```python
from build123d import *

# Parameters (mm, degrees)
SKETCH2_R          = 4
SKETCH2_R_2        = 1.75
CUT_EXTRUDE1_DEPTH = 21.310096012


with BuildPart() as part:
    # Sketch1 → Revolve1 (revolve)
    with BuildSketch(Plane.XY, mode=Mode.PRIVATE) as revolve1_sk:
        Polygon((0, 0), (12.5, 0), (12.5, -4), (6.5, -4), (6.5, -10), (0, -10), align=None)
    revolve(revolve1_sk.sketch.rotate(Axis((0, -10, 0), (0, 1, 0)), 90), axis=Axis((0, -10, 0), (0, 1, 0)))

    # Sketch2 → Cut-Extrude1 (cut, through all)
    with BuildSketch(Plane(origin=(0, 0, 0), x_dir=(1, 0, 0), z_dir=(0, 1, 0))):
        with Locations(Location((0, 0, 0), (0, 0, 270))):
            Circle(SKETCH2_R)
        with Locations(Location((0, 9.5, 0), (0, 0, 270))):
            Circle(SKETCH2_R_2)
        with Locations(Location((9.5, 0, 0), (0, 0, 270))):
            Circle(SKETCH2_R_2)
        with Locations(Location((0, -9.5, 0), (0, 0, 270))):
            Circle(SKETCH2_R_2)
        with Locations(Location((-9.5, 0, 0), (0, 0, 270))):
            Circle(SKETCH2_R_2)
    extrude(amount=-CUT_EXTRUDE1_DEPTH, mode=Mode.SUBTRACT)


solid = part.part
```
Check sheet for the modelled part. Datum: model origin and axes. Units: mm. A direction names the side the tool comes from. Give positions to 0.01 mm unless a question says otherwise; leave off trailing zeros. Order: outer loops, then holes, each group sorted by start corner. A loop starts at its lowest first (then second) coordinate and runs counter-clockwise, first axis right, second up. Notation, with made-up numbers: M -18,11.5 L 36,11.5 A9 cw 36,16.5 Z; hole C 72,15 d4. An arc over 180 degrees is marked long. Answer in a Markdown table with one row per item. Add a question column.
Q1. Sectioned sample at D-D, the plane z = -9.5. Record the boundary of the cut face in (x, y), and give its area (3 significant figures).
Q2. Sectioned sample at A-A, the plane x = 0. Record the boundary of the cut face in (y, z), and give its area (3 significant figures).
Q3. Thickness scan on L1, parallel to X at y = -0.25, z = 0; L2, parallel to X at y = -8, z = -0.25; L3, parallel to Y at x = 9.25, z = 3.25. Record the ranges inside material, lowest first.
Q4. Sectioned sample at C-C, the plane x = 10.25. Record the boundary of the cut face in (y, z).
Q5. Gauge pin test, flat ends, axial feed: pin 1 Ø5 at (y, z) = (-4.5, -5) entering from +X; pin 2 Ø5 at (x, z) = (0, 0) entering from -Y (3 decimals); pin 3 Ø4.5 at (x, z) = (0, 9.5) entering from -Y; pin 4 Ø5 at (x, y) = (-5, -5.5) entering from +Z. Record the tip position at first contact, or that the pin passes through.
Q6. Release check for a two-part mould opening along Z. For faces 1 (the cylindrical face through (-3.755, -2.028, -11.923)), 2 (the cylindrical face through (-3.905, -4.93, -0.867)), 3 (the flat face through (-3, -10, -3)) record: released by +Z, released by -Z, zero draft, split by the parting line, or undercut.
Q7. Sectioned sample at B-B, the plane z = 0. Record the boundary of the cut face in (x, y).
Q8. Access from +Z, -Z, +X, -X, +Y, -Y to the whole of each face (thin tool, end or side, straight path). Record for faces 4 (the cylindrical face through (0.526, -1.972, 11.169)), 5 (the cylindrical face through (3.955, -7.042, 5.158)).
Verdict:
| question | item | result |
|---|---|---|
| 1 | outline | M -8.12,-4 L -1.75,-4 L -1.75,0 L -8.12,0 Z; M 1.75,-4 L 8.12,-4 L 8.12,0 L 1.75,0 Z |
| 1 | area | 51.0 mm² |
| 2 | outline | M -10,-6.5 L -4,-6.5 L -4,-7.75 L 0,-7.75 L 0,-4 L -10,-4 Z; M -10,4 L 0,4 L 0,7.75 L -4,7.75 L -4,6.5 L -10,6.5 Z; M -4,-12.5 L 0,-12.5 L 0,-11.25 L -4,-11.25 Z; M -4,11.25 L 0,11.25 L 0,12.5 L -4,12.5 Z |
| 2 | area | 70.0 mm² |
| 3 | L1 | -12.5 to -11.25, -7.75 to -4, 4 to 7.75, 11.25 to 12.5 |
| 3 | L2 | -6.5 to -3.99, 3.99 to 6.5 |
| 3 | L3 | -4 to 0 |
| 4 | outline | M -4,-7.15 L 0,-7.15 L 0,-1.58 L -4,-1.58 Z; M -4,1.58 L 0,1.58 L 0,7.15 L -4,7.15 Z |
| 5 | pin 1 | x = 12.24 |
| 5 | pin 2 | through |
| 5 | pin 3 | y = -4 |
| 5 | pin 4 | z = 12.13 |
| 6 | face 1 | split by the parting line |
| 6 | face 2 | undercut |
| 6 | face 3 | zero draft |
| 7 | outline | M -12.5,-4 L -11.25,-4 L -11.25,0 L -12.5,0 Z; M -7.75,-4 L -6.5,-4 L -6.5,-10 L -4,-10 L -4,0 L -7.75,0 Z; M 4,-10 L 6.5,-10 L 6.5,-4 L 7.75,-4 L 7.75,0 L 4,0 Z; M 11.25,-4 L 12.5,-4 L 12.5,0 L 11.25,0 Z |
| 8 | face 4 | +Y, -Y |
| 8 | face 5 | -Y |
